Could you check a few things on this model? Use its own coordinates, in mm. A direction names the side the tool comes from. Round coordinates to 2 decimals unless told otherwise and drop trailing zeros. Loops run counter-clockwise (first coordinate to the right, second up) from the corner with the lowest first, then second, coordinate; pieces in that order, holes last.
from build123d import *

# Parameters (mm, degrees)
BOSS_EXTRUDE1_DEPTH     = 50
CUT_EXTRUDE1_DEPTH      = 56.012411105
CUT_EXTRUDE1_DEPTH_BACK = 56.012411105
SKETCH3_R               = 11.25
CUT_EXTRUDE2_DEPTH      = 7
CUT_EXTRUDE3_DEPTH      = 24
CUT_EXTRUDE3_DEPTH_BACK = 3
SKETCH5_R               = 2
CUT_EXTRUDE4_DEPTH      = 56.012411105
CUT_EXTRUDE4_DEPTH_BACK = 56.012411105
CUT_EXTRUDE5_DEPTH      = 3
CUT_EXTRUDE5_DEPTH_BACK = 15
SKETCH7_R               = 2.5
CUT_EXTRUDE7_DEPTH      = 10
CUT_EXTRUDE7_DEPTH_BACK = 1
CUT_EXTRUDE8_DEPTH      = 10
SKETCH11_R              = 2.1
CUT_EXTRUDE9_DEPTH      = 10
SKETCH12_R              = 5
CUT_EXTRUDE10_DEPTH     = 1.5


with BuildPart() as part:
    # Sketch1 → Boss-Extrude1 (new body)
    with BuildSketch(Plane.XY):
        with BuildLine():
            Line((-11.66190379, -15), (11.66190379, -15))
            ThreePointArc((11.66190379, -15), (13.435028843, -13.435028843), (15, -11.66190379))
            ThreePointArc((15, -11.66190379), (17.359878328, 0), (15, 11.66190379))
            ThreePointArc((15, 11.66190379), (13.435028843, 13.435028843), (11.66190379, 15))
            Line((11.66190379, 15), (-11.66190379, 15))
            ThreePointArc((-11.66190379, 15), (-13.435028843, 13.435028843), (-15, 11.66190379))
            ThreePointArc((-15, 11.66190379), (-17.359878328, 0), (-15, -11.66190379))
            ThreePointArc((-15, -11.66190379), (-13.435028843, -13.435028843), (-11.66190379, -15))
        make_face()
    extrude(amount=BOSS_EXTRUDE1_DEPTH)

    # Sketch2 → Cut-Extrude1 (cut, two sides: drawn at the far end of the back side and taken through both)
    with BuildSketch(Plane(origin=(0, 0, 0), x_dir=(1, 0, 0), z_dir=(0, 1, 0)).offset(-CUT_EXTRUDE1_DEPTH_BACK)):
        with BuildLine():
            Line((-11, -35), (-11, -50))
            Line((-11, -50), (11, -50))
            Line((11, -50), (11, -35))
            ThreePointArc((11, -35), (0, -24), (-11, -35))
        make_face()
    extrude(amount=CUT_EXTRUDE1_DEPTH + CUT_EXTRUDE1_DEPTH_BACK, mode=Mode.SUBTRACT)

    # Sketch3 → Cut-Extrude2 (cut)
    with BuildSketch(Plane(origin=(0, 0, 0), x_dir=(-1, 0, 0), z_dir=(0, 0, -1))):
        Circle(SKETCH3_R)
    extrude(amount=-CUT_EXTRUDE2_DEPTH, mode=Mode.SUBTRACT)

    # Sketch4 → Cut-Revolve1 (revolve, cut)
    with BuildSketch(Plane(origin=(0, 0, 0), x_dir=(1, 0, 0), z_dir=(0, 1, 0)), mode=Mode.PRIVATE) as cut_revolve1_sk:
        Polygon((0, -7), (9, -7), (0, -9), align=None)
    revolve(cut_revolve1_sk.sketch.rotate(Axis((0, 0, 9), (0, 0, -1)), 180), axis=Axis((0, 0, 9), (0, 0, -1)), mode=Mode.SUBTRACT)

    # Sketch5 → Cut-Extrude3 (cut, two sides: drawn at the far end of the back side and taken through both)
    with BuildSketch(Plane.ZY.offset(-11).offset(-CUT_EXTRUDE3_DEPTH_BACK)):
        with Locations((43, 0)):
            Circle(SKETCH5_R)
    extrude(amount=CUT_EXTRUDE3_DEPTH + CUT_EXTRUDE3_DEPTH_BACK, mode=Mode.SUBTRACT)

    # Sketch6 → Cut-Extrude4 (cut, two sides: drawn at the far end of the back side and taken through both)
    with BuildSketch(Plane(origin=(0, 0, 0), x_dir=(1, 0, 0), z_dir=(0, 1, 0)).offset(-CUT_EXTRUDE4_DEPTH_BACK)):
        Polygon((0, -24), (-19.504315736, -4.495684264), (-19.504315736, 1.223091499), (17.994194722, 1.223091499), (17.994194722, -52.44895982), (0, -52.44895982), align=None)
    extrude(amount=CUT_EXTRUDE4_DEPTH + CUT_EXTRUDE4_DEPTH_BACK, mode=Mode.SUBTRACT)

    # Sketch7 → Cut-Extrude5 (cut, two sides: drawn at the far end of the back side and taken through both)
    with BuildSketch(Plane(origin=(0, 0, 0), x_dir=(0, 0, -1), z_dir=(1, 0, 0)).offset(-CUT_EXTRUDE5_DEPTH_BACK)):
        with Locations((-18, 6)):
            Circle(SKETCH7_R)
        with Locations(Location((-18, -6, 0), (0, 0, 180))):
            Circle(SKETCH7_R)
    extrude(amount=CUT_EXTRUDE5_DEPTH + CUT_EXTRUDE5_DEPTH_BACK, mode=Mode.SUBTRACT)

    # Sketch9 → Cut-Extrude7 (cut, two sides: drawn at the far end of the back side and taken through both)
    with BuildSketch(Plane.ZY.offset(15).offset(-CUT_EXTRUDE7_DEPTH_BACK)):
        with BuildLine():
            Line((13, 6), (13, -6))
            ThreePointArc((13, -6), (18, -11), (23, -6))
            Line((23, -6), (23, 6))
            ThreePointArc((23, 6), (18, 11), (13, 6))
        make_face()
    extrude(amount=CUT_EXTRUDE7_DEPTH + CUT_EXTRUDE7_DEPTH_BACK, mode=Mode.SUBTRACT)

    # Sketch10 → Cut-Extrude8 (cut)
    with BuildSketch(Plane(origin=(-11, 0, 0), x_dir=(0, 0, -1), z_dir=(1, 0, 0))):
        with BuildLine():
            Line((-35, 15), (-35, 16.580470579))
            Line((-35, 16.580470579), (-52.035721035, 16.580470579))
            Line((-52.035721035, 16.580470579), (-52.035721035, -15.90001351))
            Line((-52.035721035, -15.90001351), (-35, -15.90001351))
            Line((-35, -15.90001351), (-35, -15))
            ThreePointArc((-35, -15), (-50, 0), (-35, 15))
        make_face()
    extrude(amount=-CUT_EXTRUDE8_DEPTH, mode=Mode.SUBTRACT)

    # Sketch11 → Cut-Extrude9 (cut)
    with BuildSketch(Plane(origin=(-11, 0, 0), x_dir=(0, 0, -1), z_dir=(1, 0, 0))):
        with Locations((-43, 0)):
            Circle(SKETCH11_R)
    extrude(amount=-CUT_EXTRUDE9_DEPTH, mode=Mode.SUBTRACT)

    # Sketch12 → Cut-Extrude10 (cut)
    with BuildSketch(Plane(origin=(-11, 0, 0), x_dir=(0, 0, -1), z_dir=(1, 0, 0))):
        with Locations((-43, 0)):
            Circle(SKETCH12_R)
    extrude(amount=-CUT_EXTRUDE10_DEPTH, mode=Mode.SUBTRACT)


solid = part.part
Item 1: If we section it at A-A, the plane y = 0: Please give me the cut outline in (x, z), then the cut area to 3 significant figures.
Results list:
outline: (-17.36, 6.64) - (0, 24) arc R11 cw to (-11, 35) - (-11, 38) - (-12.5, 38) - (-12.5, 40.9) - (-17.36, 40.9) - (-17.36, 23) - (-14, 23) - (-14, 13) - (-17.36, 13) - close; (-17.36, 45.1) - (-12.5, 45.1) - (-12.5, 48) - (-11, 48) - (-11, 50) - (-17.36, 50) - close
area: 273 mm2
Item 2: If we section it at C-C, the plane z = 43: Please give me the cut outline in (x, y).
Results list:
outline: (-17.29, -2.1) arc R29.99 ccw to (-15, -11.66) arc R19 ccw to (-14.14, -12.69) - (-11, -12.69) - (-11, -5) - (-12.5, -5) - (-12.5, -2.1) - close; (-17.29, 2.1) - (-12.5, 2.1) - (-12.5, 5) - (-11, 5) - (-11, 12.69) - (-14.14, 12.69) arc R19 ccw to (-15, 11.66) arc R29.99 ccw to start
Item 3: If I drill on line 1 along Y through (x, z) = (-6.25, 18); line 2 along Z through (x, y) = (-15.5, -3); line 3 along Z through (x, y) = (-13.9, 0), over which ranges is the centre line in solid material (lowest first)?
Results list:
line 1: y = -15 to -8.5, -3.5 to 3.5, 8.5 to 15
line 2: z = 8.5 to 13, 23 to 49.7
line 3: z = 10.1 to 40.9, 45.1 to 50
Item 4: We'd pull the mould along Y, two halves only. Please class faces 1 (the cylindrical face through (-17.36, 0.17, 32.64)), 2 (the flat face through (-16, 0, 13)), 3 (the flat face through (-9, -15, 24)): released by +Y, released by -Y, zero draft, split by the parting line, or undercut.
Results list:
face 1: split by the parting line
face 2: undercut
face 3: released by -Y
Item 5: For faces 4 (the cylindrical face through (-15, 11, 18)), 5 (the flat face through (-11, 0, 37)), 6 (the flat face through (-12.5, -1, 40.8)), which set-ups out of +Z, -Z, +X, -X, +Y, -Y let a thin tool reach every point of the face, with its end or its side?
Results list:
face 4: -X
face 5: +Z, +X, +Y, -Y
face 6: +X
Item 6: If we section it at D-D, the plane z = 18: Please give me the cut outline in (x, y), then the cut area to 3 significant figures.
Results list:
outline: (-15.27, -11) arc R29.99 ccw to (-15, -11.66) arc R19 ccw to (-11.66, -15) - (-6, -15) - (-6, -8.5) - (-14, -8.5) - (-14, -11) - close; (-15.27, 11) - (-14, 11) - (-14, 8.5) - (-6, 8.5) - (-6, 15) - (-11.66, 15) arc R19 ccw to (-15, 11.66) arc R29.99 ccw to start; (-14, -3.5) - (-6, -3.5) - (-6, 3.5) - (-14, 3.5) - close
area: 158 mm2
Item 7: Will these pins go through, and if not, where does the flat tip stop? pin 1 (12 mm diameter, centred on y = -9, z = 33, fed in from -X); pin 2 (6 mm diameter, centred on y = 0, z = 43, fed in from +X); pin 3 (1.5 mm diameter, centred on x = -8, z = 15, fed in from +Y); pin 4 (1.5 mm diameter, centred on x = -4, y = 6.5, fed in from -Z).
Results list:
pin 1: stops at x = -17.21
pin 2: stops at x = -12.5
pin 3: stops at y = 15
pin 4: stops at z = 20.17
Item 8: If we section it at B-B, the plane x = -16: Please give me the cut outline in (y, z), then the cut area to 3 significant figures.
Results list:
outline: (-8.93, 8) - (8.93, 8) - (8.93, 13.95) arc R5 cw to (6, 13) - (-6, 13) arc R5 cw to (-8.93, 13.95) - close; (-8.93, 22.05) arc R5 cw to (-6, 23) - (6, 23) arc R5 cw to (8.93, 22.05) - (8.93, 47.05) arc R15 ccw to (-8.93, 47.05) - close; hole circle Ø4.2 at (0, 43)
area: 544 mm2
